from build123d import *

# Parameters (mm, degrees)
F2_R            = 4.5
F3_DEPTH        = 46
F1_R            = 5
F4_DEPTH        = 30
F0_R            = 8
F5_DEPTH        = 16
F6_SIZE2        = 1.5
F6_SIZE         = 1.5
F7_SIZE2        = 0.49999
F7_SIZE         = 0.49999
F8_SIZE2        = 0.5
F8_SIZE         = 0.5
F10_DEPTH       = 3
F12_D           = 3.4
F12_CSINK_D     = 6.3
F12_CSINK_ANGLE = 90
F13_D           = 3.4
F13_CSINK_D     = 6.3
F13_CSINK_ANGLE = 90
F15_R           = 0.5


# Not quite as in the source:
# - a fillet or chamfer is up to 0.001 mm smaller than in the source, because OpenCascade refuses the exact size
# - a feature of the source that left no trace in its solid (it failed there, or was rolled back) is left out


with BuildPart() as f3:
    # F2 (on Top) → F3 (new body)
    with BuildSketch(Plane.XY):
        Circle(F2_R)
    extrude(amount=-F3_DEPTH)

    # F1 (on Top) → F4 (join)
    with BuildSketch(Plane.XY):
        Circle(F1_R)
    extrude(amount=-F4_DEPTH)

    # F0 (on Top) → F5 (join)
    with BuildSketch(Plane.XY):
        Circle(F0_R)
    extrude(amount=-F5_DEPTH)

    # F6
    f6_edges = [f3.edges().sort_by_distance(p)[0] for p in [
        (-4.5, 0, -46),
    ]]
    chamfer(f6_edges, length=F6_SIZE, length2=F6_SIZE2)

    # F7 (size 0.5 and 0.5 in the source; OpenCascade refuses exactly that, so slightly less here)
    f7_edges = [f3.edges().sort_by_distance(p)[0] for p in [
        (-5, 0, -30),
    ]]
    chamfer(f7_edges, length=F7_SIZE, length2=F7_SIZE2)

    # F8
    f8_edges = [f3.edges().sort_by_distance(p)[0] for p in [
        (-8, 0, -16),
    ]]
    chamfer(f8_edges, length=F8_SIZE, length2=F8_SIZE2)

    # F9 (on Top) → F10 (join)
    with BuildSketch(Plane.XY):
        with BuildLine():
            Line((11.1242977306, 8.5), (-11.1242977306, 8.5))
            ThreePointArc((-11.1242977306, 8.5), (-14, 0), (-11.1242977306, -8.5))
            Line((-11.1242977306, -8.5), (11.1242977306, -8.5))
            ThreePointArc((11.1242977306, -8.5), (14, 0), (11.1242977306, 8.5))
        make_face()
    extrude(amount=-F10_DEPTH)

    # F12 (through all)
    with Locations(Plane.XY):
        with Locations((-10, 0)):
            CounterSinkHole(F12_D / 2, F12_CSINK_D / 2, counter_sink_angle=F12_CSINK_ANGLE)

    # F13 (through all)
    with Locations(Plane.XY):
        with Locations((10, 0)):
            CounterSinkHole(F13_D / 2, F13_CSINK_D / 2, counter_sink_angle=F13_CSINK_ANGLE)

    # F15
    f15_edges = [f3.edges().sort_by_distance(p)[0] for p in [
        (-5, 0, -16),
    ]]
    fillet(f15_edges, radius=F15_R)


solid = f3.part
CAD build for the part. Positions are in the model's coordinates, mm. A direction names the side the tool comes from. Round coordinates to 2 decimals unless told otherwise and drop trailing zeros. Loops run counter-clockwise (first coordinate to the right, second up) from the corner with the lowest first, then second, coordinate; pieces in that order, holes last. Notation, with made-up numbers: (28, 23.25) - (70, 23.25) arc R11 ccw to (70, 39.25) - close; hole circle Ø5 at (-30, 40.25). An arc over 180 degrees is marked (long way). Put each result on its own line as item: value.
1. Pin check, flat tips, straight feed: P1, Ø6, axis at x = -4, z = -28.5, coming from the -Y side; P2, Ø12, axis at x = 2, z = -18, coming from the -Y side; P3, Ø4, axis at y = -0.5, z = -32.5, coming from the -X side. Stop position of each tip, or through.
Geometry check:
P1: y = -4.9
P2: y = -8
P3: x = -4.5
2. Slice it at A-A on x = -10. List the corners of the cut face in (y, z), and give its area (3 significant figures).
Geometry check:
outline: (-8.5, -3) - (-1.7, -3) - (-1.7, -1.45) - (-3.15, 0) - (-8.5, 0) - close; (1.7, -3) - (8.5, -3) - (8.5, 0) - (3.15, 0) - (1.7, -1.45) - close
area: 38.7 mm²
3. Slice it at C-C on y = 0. Give the number of separate pieces and of enclosed holes in the cut face, and give its area (3 significant figures).
Geometry check:
separate pieces: 3
enclosed holes: 0
area: 549 mm²
4. Wall check: line 1 (Y direction, x = -10, z = -1.9); line 2 (X direction, y = 0, z = -2.55); line 3 (X direction, y = 2.75, z = -11). Give the ranges that are in metal, low to high.
Geometry check:
line 1: -8.5 to -1.7, 1.7 to 8.5
line 2: -14 to -11.7, -8.3 to 8.3, 11.7 to 14
line 3: -7.51 to 7.51
5. 3-axis set-ups, long thin cutter, end or side, ignore diameter. For faces 1 (the flat face through (-4, 4, -16)), 2 (the cylindrical face through (8.43, -0.65, -2.24)): which of +Z, -Z, +X, -X, +Y, -Y reach the whole face in a straight line?
Geometry check:
face 1: -Z
face 2: +Z, -Z
6. Slice it at D-D on z = -39. List the corners of the cut face in (x, y).
Geometry check:
outline: circle Ø9 at (0, 0)
